Can you work these out from the model? Positions are in its coordinate system, mm. Give positions to 0.01 mm unless a question says otherwise; leave off trailing zeros. Write each loop counter-clockwise with the first axis right and the second up, starting at its lowest first coordinate (ties: lowest second). Pieces come first, ordered by that corner, then holes.
1. Suppose I cut it at A-A (y = 0). Please give me the cut outline in (x, z).
2. I'm going to push a flat-ended pin straight in: pin 1 (6 mm diameter, centred on x = -82.55, y = 0, fed in from +Z). Where does the tip first touch, or does it pass through?
3. If I drill on probe 1 along Y at (x, z) = (-82.55, -2.75); probe 2 along X at (y, z) = (0, -2.75); probe 3 along X at (y, z) = (1.25, -2.25), over which ranges is the centre line in solid material (lowest first)?
4. Suppose I cut it at B-B (x = -82.55). Please give me the cut outline in (y, z).
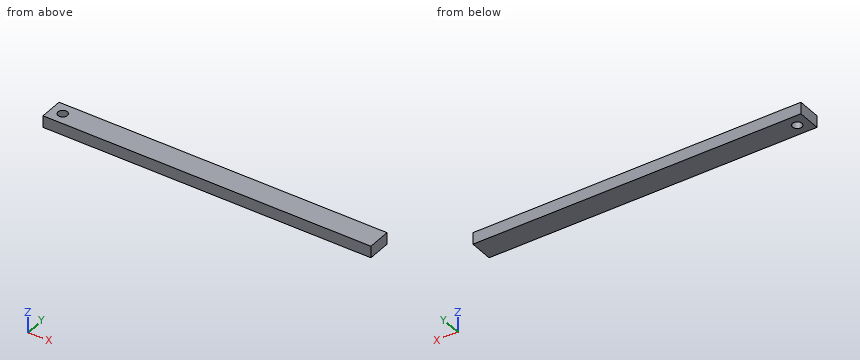
Autodesk Inventor part; units mm, degrees
ref_plane "YZ Plane" through (0, 0, 0) normal (1, 0, 0) x (0, 1, 0)
ref_plane "XZ Plane" through (0, 0, 0) normal (0, 1, 0) x (-1, 0, 0)
ref_plane "XY Plane" through (0, 0, 0) normal (0, 0, 1) x (1, 0, 0)
sketch "Sketch1" plane through (0, 0, 0) normal (0, 0, 1) x (1, 0, 0)
  line L0 (-88.9, -6.35) -> (88.9, -6.35)
  line L1 (88.9, -6.35) -> (88.9, 6.35)
  line L2 (88.9, 6.35) -> (-88.9, 6.35)
  line L3 (-88.9, 6.35) -> (-88.9, -6.35)
  line L4 (-88.9, -6.35) -> (88.9, 6.35) construction
  line L5 (88.9, -6.35) -> (-88.9, 6.35) construction
  point P0 (0, 0)
  point P1 (-82.55, 0)
  dimension "d0" = 177.8
  dimension "d1" = 12.7
  dimension "d2" = 6.35
extrude "Extrusion1" add sketch "Sketch1" against normal blind 6.35
hole "Hole1" at (-82.55, 0, 0) direction (0, 0, -1) diameter 5.1054 end through all
properties part number "CL6-007" material "Aluminum 6061"
Checks:
1. outline: (-88.9, -6.35) - (-85.1, -6.35) - (-85.1, 0) - (-88.9, 0) - close; (-80, -6.35) - (88.9, -6.35) - (88.9, 0) - (-80, 0) - close
2. pin 1: stops at z = 0
3. probe 1: y = -6.35 to -2.55, 2.55 to 6.35
3. probe 2: x = -88.9 to -85.1, -80 to 88.9
3. probe 3: x = -88.9 to -84.78, -80.32 to 88.9
4. outline: (-6.35, -6.35) - (-2.55, -6.35) - (-2.55, 0) - (-6.35, 0) - close; (2.55, -6.35) - (6.35, -6.35) - (6.35, 0) - (2.55, 0) - close
